Solid Edge part; units mm, degrees
sketch "Sketch1" plane through (0, 0, 0) normal (0, -1, 0) x (1, 0, 0)
  line L0 (40, -27) -> (40, 27)
  line L1 (40, 27) -> (-40, 27)
  line L2 (-40, 27) -> (-40, -27)
  line L3 (-40, -27) -> (40, -27)
extrude "Protrusion1" add sketch "Sketch1" along normal blind 2
sketch "Sketch2" plane through (0, 0, 0) normal (0, -1, 0) x (1, 0, 0)
  line L0 (-25, 23) -> (-15, 23)
  line L1 (-15, 23) -> (-15, 25)
  line L2 (-15, 25) -> (-25, 25)
  line L3 (-25, 25) -> (-25, 23)
extrude "ExtrudedCutout_1" cut sketch "Sketch2" along normal blind 2
sketch "Sketch3" plane through (0, 0, 0) normal (0, -1, 0) x (1, 0, 0)
  line L0 (25, 25) -> (15, 25)
  line L1 (15, 25) -> (15, 23)
  line L2 (15, 23) -> (25, 23)
  line L3 (25, 23) -> (25, 25)
extrude "ExtrudedCutout_2" cut sketch "Sketch3" along normal blind 2
sketch "Sketch4" plane through (0, 0, 0) normal (0, -1, 0) x (1, 0, 0)
  line L0 (15, -25) -> (25, -25)
  line L1 (25, -25) -> (25, -23)
  line L2 (25, -23) -> (15, -23)
  line L3 (15, -23) -> (15, -25)
extrude "ExtrudedCutout_3" cut sketch "Sketch4" along normal blind 2
sketch "Sketch5" plane through (0, 0, 0) normal (0, -1, 0) x (1, 0, 0)
  line L0 (-15, -23) -> (-25, -23)
  line L1 (-25, -23) -> (-25, -25)
  line L2 (-25, -25) -> (-15, -25)
  line L3 (-15, -25) -> (-15, -23)
extrude "ExtrudedCutout_4" cut sketch "Sketch5" along normal blind 2
sketch "Sketch6" plane through (0, 0, 0) normal (0, -1, 0) x (1, 0, 0)
  line L0 (-38, -27) -> (-38, -5)
  line L1 (-38, -5) -> (-40, -5)
  line L2 (-40, -5) -> (-40, -27)
  line L3 (-40, -27) -> (-38, -27)
extrude "ExtrudedCutout_5" cut sketch "Sketch6" along normal blind 2
sketch "Sketch7" plane through (0, 0, 0) normal (0, -1, 0) x (1, 0, 0)
  line L0 (-38, 5) -> (-38, 27)
  line L1 (-38, 27) -> (-40, 27)
  line L2 (-40, 27) -> (-40, 5)
  line L3 (-40, 5) -> (-38, 5)
extrude "ExtrudedCutout_6" cut sketch "Sketch7" along normal blind 2
sketch "Sketch8" plane through (0, 0, 0) normal (0, -1, 0) x (1, 0, 0)
  line L0 (38, -5) -> (38, -27)
  line L1 (38, -27) -> (40, -27)
  line L2 (40, -27) -> (40, -5)
  line L3 (40, -5) -> (38, -5)
extrude "ExtrudedCutout_7" cut sketch "Sketch8" along normal blind 2
sketch "Sketch9" plane through (0, 0, 0) normal (0, -1, 0) x (1, 0, 0)
  line L0 (38, 27) -> (38, 5)
  line L1 (38, 5) -> (40, 5)
  line L2 (40, 5) -> (40, 27)
  line L3 (40, 27) -> (38, 27)
extrude "ExtrudedCutout_8" cut sketch "Sketch9" along normal blind 2
sketch "Sketch10" plane through (0, 0, 0) normal (0, -1, 0) x (1, 0, 0)
  line L0 (-20.12, -1) -> (-6.12, -1)
  line L1 (-6.12, -1) -> (-6.12, 8)
  line L2 (-6.12, 8) -> (-20.12, 8)
  line L3 (-20.12, 8) -> (-20.12, -1)
extrude "ExtrudedCutout_9" cut sketch "Sketch10" along normal blind 2
properties material "Acrylic, high impact grade"
Check sheet for the modelled part. Datum: model origin and axes. Units: mm. A direction names the side the tool comes from. Round coordinates to 2 decimals unless told otherwise and drop trailing zeros. Loops run counter-clockwise (first coordinate to the right, second up) from the corner with the lowest first, then second, coordinate; pieces in that order, holes last. Notation, with made-up numbers: M -8,-26 L 3,-26 A21 ccw 3,-11 Z; hole C -39,11.5 d5. An arc over 180 degrees is marked long. Answer as a JSON object with one key per item and string values.
1. Section check B-B (x = 19). Record the boundary of the cut face in (y, z), plus the area to 3 significant figures.
Reply:
{"outline": "M -2,-27 L 0,-27 L 0,-25 L -2,-25 Z; M -2,-23 L 0,-23 L 0,23 L -2,23 Z; M -2,25 L 0,25 L 0,27 L -2,27 Z", "area": "100 mm²"}
2. Mould release check, pull along X, two halves, no side actions. Record for faces 6 (the flat face through (-20, -1, -23)), 7 (the flat face through (-40, -1, 0)), 8 (the flat face through (-6.12, -1, 3)), 9 (the flat face through (-1, -1, -27)): pulls with the +X half, pulls with the -X half, needs draft (parallel to the pull), parting line crosses it, or undercut.
Reply:
{"face 6": "undercut", "face 7": "pulls with the -X half", "face 8": "undercut", "face 9": "needs draft"}
3. Access from +Z, -Z, +X, -X, +Y, -Y to the whole of each face (thin tool, end or side, straight path). Record for faces 1 (the flat face through (-38, -1, 16)), 2 (the flat face through (25, -1, -24)), 3 (the flat face through (1, -2, 0)), 4 (the flat face through (38, -1, 16)), 5 (the flat face through (-39, -1, -5)).
Reply:
{"face 1": "+Z, -X, +Y, -Y", "face 2": "+Y, -Y", "face 3": "+Z, -Z, +X, -X, -Y", "face 4": "+Z, +X, +Y, -Y", "face 5": "-Z, -X, +Y, -Y"}
4. Scan lines: line 1 (Z direction, x = -17, y = -0.8); line 2 (Z direction, x = -21, y = -1.45); line 3 (Z direction, x = -8, y = -0.5). Record each from-to range of solid material in increasing order.
Reply:
{"line 1": "z = -27 to -25, -23 to -1, 8 to 23, 25 to 27", "line 2": "z = -27 to -25, -23 to 23, 25 to 27", "line 3": "z = -27 to -1, 8 to 27"}
5. Section check C-C (z = 7). Record the boundary of the cut face in (x, y), plus the area to 3 significant figures.
Reply:
{"outline": "M -38,-2 L -20.12,-2 L -20.12,0 L -38,0 Z; M -6.12,-2 L 38,-2 L 38,0 L -6.12,0 Z", "area": "124 mm²"}
6. Section check A-A (x = -18). Record the boundary of the cut face in (y, z).
Reply:
{"outline": "M -2,-27 L 0,-27 L 0,-25 L -2,-25 Z; M -2,-23 L 0,-23 L 0,-1 L -2,-1 Z; M -2,8 L 0,8 L 0,23 L -2,23 Z; M -2,25 L 0,25 L 0,27 L -2,27 Z"}
7. Gauge pin test, flat ends, axial feed: P1, Ø1, axis at y = -1, z = -24.5, coming from the -X side; P2, Ø0.6, axis at x = -39, y = -1.5, coming from the -Z side. Record the tip position at first contact, or that the pin passes through.
Reply:
{"P1": "stops at x = -38", "P2": "stops at z = -5"}
8. Section check D-D (y = -0.4). State how many separate pieces and enclosed holes the cut face has, plus the area to 3 significant figures.
Reply:
{"separate pieces": "1", "enclosed holes": "5", "area": "3,940 mm²"}
